Geometry check sheet. Reference: the model listing, model coordinates, mm. Coordinates: 2 decimals unless noted, no trailing zeros. Use CSV: the item, a comma, the result in double quotes. Start each with the question number.
```python
from build123d import *

# Parameters (mm, degrees)
F0_R     = 3
F1_DEPTH = 3


with BuildPart() as f1:
    # F0 (on Top) → F1 (new body)
    with BuildSketch(Plane.XY):
        with BuildLine():
            ThreePointArc((35.620954, -8.242963), (36.326171, -4.148268), (36.562259, 0))
            ThreePointArc((36.562259, 0), (35.106793, 10.213321), (30.85627, 19.613501))
            Line((30.85627, 19.613501), (13.104219, 19.613501))
            Line((13.104219, 19.613501), (18.847004, 31.330325))
            ThreePointArc((18.847004, 31.330325), (5.274088, 36.179867), (-9.118436, 35.406962))
            Line((-9.118436, 35.406962), (-14.604121, 18.523758))
            Line((-14.604121, 18.523758), (-23.972865, 27.606169))
            ThreePointArc((-23.972865, 27.606169), (-32.779316, 16.196149), (-36.491773, 2.269205))
            Line((-36.491773, 2.269205), (-22.130062, -8.165189))
            Line((-22.130062, -8.165189), (-33.663049, -14.268774))
            ThreePointArc((-33.663049, -14.268774), (-25.532819, -26.170097), (-13.43472, -34.004516))
            Line((-13.43472, -34.004516), (0.926991, -23.570122))
            Line((0.926991, -23.570122), (3.167956, -36.424756))
            ThreePointArc((3.167956, -36.424756), (16.999166, -32.370159), (28.188659, -23.285152))
            Line((28.188659, -23.285152), (22.702974, -6.401948))
            Line((22.702974, -6.401948), (35.620954, -8.242963))
        make_face()
        Polygon((-16.89326, -11.515298), (-10.23678, -15.379139), (-10.254725, -23.07574), (-16.92915, -26.9085), (-23.58563, -23.044659), (-23.567685, -15.348058), align=None, mode=Mode.SUBTRACT)
        Polygon((5.731394, -19.624868), (11.463091, -14.488172), (18.777449, -16.883619), (20.36011, -24.415762), (14.628413, -29.552458), (7.314055, -27.157011), align=None, mode=Mode.SUBTRACT)
        Polygon((-16.172003, 12.508023), (-17.78977, 4.983341), (-25.115218, 2.622027), (-30.8229, 7.785395), (-29.205133, 15.310076), (-21.879685, 17.67139), align=None, mode=Mode.SUBTRACT)
        Circle(F0_R, mode=Mode.SUBTRACT)
        Polygon((20.435457, -0.613538), (17.32136, 6.424956), (21.859827, 12.64109), (29.51239, 11.818729), (32.626486, 4.780235), (28.08802, -1.435898), align=None, mode=Mode.SUBTRACT)
        Polygon((5.535865, 32.506806), (10.045296, 26.269577), (6.898412, 19.245681), (-0.757902, 18.459013), (-5.267333, 24.696242), (-2.12045, 31.720139), align=None, mode=Mode.SUBTRACT)
    extrude(amount=F1_DEPTH)


solid = f1.part
```
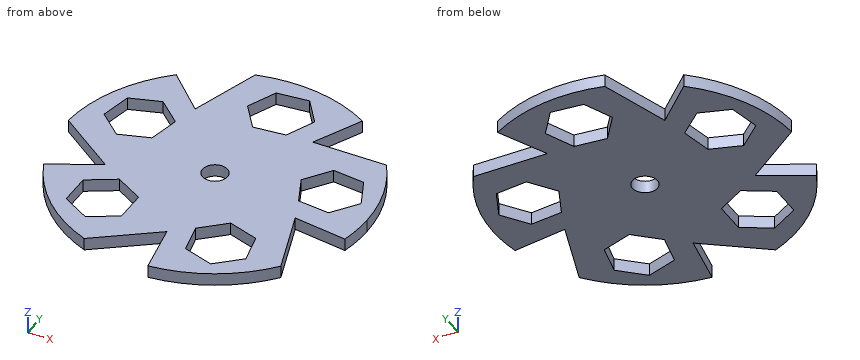
1) Section check A-A on z = 1.75. State how many separate pieces and enclosed holes the cut face has, then the cut area to 3 significant figures.
2) Gauge pin test, flat end, axial feed: P1, Ø0.9, axis at x = 23, z = 2, coming from the +Y side. Record the tip position at first contact, or that the pin passes through.
3) Material ranges on line 1 along Y through (x, z) = (-2.5, 2.4); line 2 along X through (y, z) = (23, 1.95); line 3 along Y through (x, z) = (0, 0.9), recorded low to high.
Results are:
1,separate pieces,"1"
1,enclosed holes,"6"
1,area,"2,830 mm²"
2,P1,"stops at y = 19.61"
3,line 1,"y = -26.06 to -1.66, 1.66 to 20.87, 30.87 to 36.48"
3,line 2,"x = -28.42 to -19.22, -13.15 to -4.04, 8.58 to 14.76"
3,line 3,"y = -24.24 to -3, 3 to 18.54, 31.94 to 36.56"
